```python
from build123d import *

# Parameters (mm, degrees)
F1_DEPTH = 12
F3_DEPTH = 15
F5_DEPTH = 9.8


with BuildPart() as f1:
    # F0 (on Top) → F1 (new body)
    with BuildSketch(Plane.XY):
        with BuildLine():
            Line((-20, -10), (-7.079002, -10))
            Line((-7.079002, -10), (7.079002, -10))
            Line((7.079002, -10), (20, -10))
            Line((20, -10), (20, -2.920998))
            ThreePointArc((20, -2.920998), (16.215527, 6.215527), (7.079002, 10))
            Line((7.079002, 10), (-7.079002, 10))
            ThreePointArc((-7.079002, 10), (-16.215527, 6.215527), (-20, -2.920998))
            Line((-20, -2.920998), (-20, -10))
        make_face()
    extrude(amount=F1_DEPTH)

    # F2 (on face) → F3 (join)
    with BuildSketch(Plane(origin=(0, 10, 0), x_dir=(-1, 0, 0), z_dir=(0, 1, 0))):
        with BuildLine():
            ThreePointArc((0, 0), (4.242641, 1.757359), (6, 6))
            ThreePointArc((6, 6), (4.242641, 10.242641), (0, 12))
            ThreePointArc((0, 12), (-6, 6), (0, 0))
        make_face()
    extrude(amount=F3_DEPTH)

    # F4 (on face) → F5 (join)
    with BuildSketch(Plane(origin=(0, 25, 0), x_dir=(-1, 0, 0), z_dir=(0, 1, 0))):
        Polygon((-3.9, 7.4), (-3.9, 4.6), (-1.4, 4.6), (-1.4, 2.1), (1.4, 2.1), (1.4, 4.6), (3.9, 4.6), (3.9, 7.4), (1.4, 7.4), (1.4, 9.9), (-1.4, 9.9), (-1.4, 7.4), align=None)
    extrude(amount=F5_DEPTH)


solid = f1.part
```
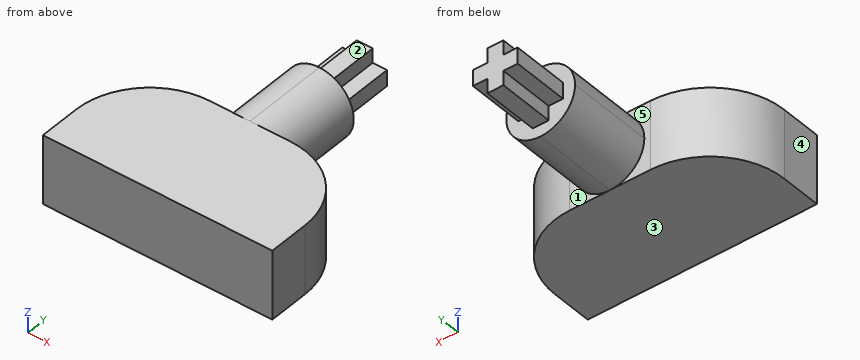
Input: part model. Units: mm. Frame: model coordinates. Face numbers are marked on the shaded views. A direction names the side the tool comes from. Give positions to 0.01 mm unless a question says otherwise; leave off trailing zeros. Order: outer loops, then holes, each group sorted by start corner. A loop starts at its lowest first (then second) coordinate and runs counter-clockwise, first axis right, second up. Notation, with made-up numbers: (26, 49.5) - (65, 49.5) arc R11 ccw to (65, 61.5) - close; hole circle Ø10 at (3.5, -33.5). An arc over 180 degrees is marked (long way). One line per item, written item: value.
1. Cut plane C-C, the plane x = 5.5. Output: boundary loops of the cut face in (y, z), and give its area (3 significant figures).
Determined:
outline: (-10, 0) - (10, 0) - (10, 3.6) - (25, 3.6) - (25, 8.4) - (10, 8.4) - (10, 12) - (-10, 12) - close
area: 312 mm2
2. Cut plane A-A, the plane y = 31. Output: boundary loops of the cut face in (x, z), and give its area (3 significant figures).
Determined:
outline: (-3.9, 4.6) - (-1.4, 4.6) - (-1.4, 2.1) - (1.4, 2.1) - (1.4, 4.6) - (3.9, 4.6) - (3.9, 7.4) - (1.4, 7.4) - (1.4, 9.9) - (-1.4, 9.9) - (-1.4, 7.4) - (-3.9, 7.4) - close
area: 35.8 mm2
3. Reachability of the marked faces 1, 2, 3, 4 and 5 from +Z, -Z, +X, -X, +Y, -Y: full face, straight path, thin tool, end or side. Return the list, or none.
Determined:
face 1: +X, +Y
face 2: +Z, +X, -X, +Y
face 3: -Z, +X, -X, +Y, -Y
face 4: +Z, -Z, -X, +Y, -Y
face 5: -X, +Y
4. Pin query (flat end, axial travel): pin 1 Ø3 at (y, z) = (29.5, 5.5) entering from -X; pin 2 Ø2 at (x, y) = (0, 28.5) entering from +Z; pin 3 Ø10 at (x, y) = (-7.5, 22) entering from -Z; pin 4 Ø1.5 at (x, y) = (1.5, 3) entering from -Z. Return the tip coordinate at first contact, or that it passes through.
Determined:
pin 1: x = -3.9
pin 2: z = 9.9
pin 3: z = 0.55
pin 4: z = 0
5. Cut plane D-D, the plane z = 3.5. Output: boundary loops of the cut face in (x, y).
Determined:
outline: (-20, -10) - (20, -10) - (20, -2.92) arc R12.92 ccw to (7.08, 10) - (5.45, 10) - (5.45, 25) - (1.4, 25) - (1.4, 34.8) - (-1.4, 34.8) - (-1.4, 25) - (-5.45, 25) - (-5.45, 10) - (-7.08, 10) arc R12.92 ccw to (-20, -2.92) - close
6. Cut plane B-B, the plane z = 10.5. Output: boundary loops of the cut face in (x, y), and give its area (3 significant figures).
Determined:
outline: (-20, -10) - (20, -10) - (20, -2.92) arc R12.92 ccw to (7.08, 10) - (3.97, 10) - (3.97, 25) - (-3.97, 25) - (-3.97, 10) - (-7.08, 10) arc R12.92 ccw to (-20, -2.92) - close
area: 847 mm2
7. Line query: probe 1 along Y at (x, z) = (1.5, 7.75); probe 2 along X at (y, z) = (28, 8); probe 3 along Z at (x, y) = (2.5, 30). Output: solid intervals per line, ascending.
Determined:
probe 1: -10 to 25
probe 2: -1.4 to 1.4
probe 3: 4.6 to 7.4
